Work out the finished part from the listing and answer in its coordinate system (mm). Give positions to 0.01 mm unless a question says otherwise; leave off trailing zeros. Write each loop counter-clockwise with the first axis right and the second up, starting at its lowest first coordinate (ties: lowest second). Pieces come first, ordered by that corner, then holes. Notation, with made-up numbers: (-13.5, 48.25) - (-2.5, 48.25) arc R16 cw to (-2.5, 57.25) - close; hole circle Ø2 at (57.5, -14.75). An arc over 180 degrees is marked (long way). Write item = value, one per line.
from build123d import *

# Parameters (mm, degrees)
SKETCH_1_W             = 295
SKETCH_1_H             = 200
EXTRUDE_1_DEPTH        = 5
SKETCH_2_R             = 1.6
CUT_EXTRUDE_549_DEPTH  = 357.440738412
SKETCH_3_R             = 1.6
CUT_EXTRUDE_902_DEPTH  = 5
SKETCH_4_R             = 1.6
CUT_EXTRUDE_1255_DEPTH = 5
SKETCH_5_R             = 1.6
CUT_EXTRUDE_1670_DEPTH = 5
SKETCH_8_R             = 1.6
CUT_EXTRUDE_2229_DEPTH = 50
SKETCH_10_R            = 1.6
CUT_EXTRUDE_2729_DEPTH = 357.440738412
CUT_EXTRUDE_3337_DEPTH = 10
FILLET_1_R             = 30


with BuildPart() as part:
    # 草图1 → 凸台-拉伸1 (new body)
    with BuildSketch(Plane.XY):
        with Locations((147.5, 100)):
            Rectangle(SKETCH_1_W, SKETCH_1_H)
    extrude(amount=EXTRUDE_1_DEPTH)

    # 草图2 → Cut-Extrude 549 (cut, through all)
    with BuildSketch(Plane.XY.offset(5)):
        with Locations((285, 120)):
            Circle(SKETCH_2_R)
        with Locations(Location((285, 80, 0), (0, 0, 180))):
            Circle(SKETCH_2_R)
    extrude(amount=-CUT_EXTRUDE_549_DEPTH, mode=Mode.SUBTRACT)

    # 草图3 → Cut-Extrude 902 (cut)
    with BuildSketch(Plane.XY.offset(5)):
        with Locations((251, 6.5)):
            Circle(SKETCH_3_R)
        with Locations((212.6, 6.5)):
            Circle(SKETCH_3_R)
        with Locations(Location((44, 6.5, 0), (0, 0, 180))):
            Circle(SKETCH_3_R)
        with Locations(Location((82.4, 6.5, 0), (0, 0, 180))):
            Circle(SKETCH_3_R)
        with Locations(Location((251, 193.5, 0), (0, 0, 180))):
            Circle(SKETCH_3_R)
        with Locations(Location((212.6, 193.5, 0), (0, 0, 180))):
            Circle(SKETCH_3_R)
        with Locations((82.4, 193.5)):
            Circle(SKETCH_3_R)
        with Locations((44, 193.5)):
            Circle(SKETCH_3_R)
    extrude(amount=-CUT_EXTRUDE_902_DEPTH, mode=Mode.SUBTRACT)

    # 草图4 → Cut-Extrude 1255 (cut)
    with BuildSketch(Plane.XY.offset(5)):
        with Locations((196, 124.5)):
            Circle(SKETCH_4_R)
        with Locations((254, 124.5)):
            Circle(SKETCH_4_R)
        with Locations((254, 75.5)):
            Circle(SKETCH_4_R)
        with Locations((196, 75.5)):
            Circle(SKETCH_4_R)
    extrude(amount=-CUT_EXTRUDE_1255_DEPTH, mode=Mode.SUBTRACT)

    # 草图5 → Cut-Extrude 1670 (cut)
    with BuildSketch(Plane.XY.offset(5)):
        with Locations((110.04, 122.5)):
            Circle(SKETCH_5_R)
        with Locations((184.96, 122.5)):
            Circle(SKETCH_5_R)
        with Locations((184.96, 77.5)):
            Circle(SKETCH_5_R)
        with Locations((110.04, 77.5)):
            Circle(SKETCH_5_R)
    extrude(amount=-CUT_EXTRUDE_1670_DEPTH, mode=Mode.SUBTRACT)

    # 草图8 → Cut-Extrude 2229 (cut)
    with BuildSketch(Plane.XY.offset(5)):
        with Locations((154.299232912, 145.494729715)):
            Circle(SKETCH_8_R)
        with Locations(Location((140.700767088, 145.494729715, 0), (0, 0, 180))):
            Circle(SKETCH_8_R)
        with Locations(Location((154.299232912, 54.505270285, 0), (0, 0, 180))):
            Circle(SKETCH_8_R)
        with Locations((140.700767088, 54.505270285)):
            Circle(SKETCH_8_R)
    extrude(amount=-CUT_EXTRUDE_2229_DEPTH, mode=Mode.SUBTRACT)

    # 草图10 → Cut-Extrude 2729 (cut, through all)
    with BuildSketch(Plane.XY.offset(5)):
        with Locations((59.36, 190.7)):
            Circle(SKETCH_10_R)
        with Locations(Location((235.64, 190.7, 0), (0, 0, 180))):
            Circle(SKETCH_10_R)
        with Locations((235.64, 9.3)):
            Circle(SKETCH_10_R)
        with Locations(Location((59.36, 9.3, 0), (0, 0, 180))):
            Circle(SKETCH_10_R)
    extrude(amount=-CUT_EXTRUDE_2729_DEPTH, mode=Mode.SUBTRACT)

    # 草图11 → Cut-Extrude 3337 (cut)
    with BuildSketch(Plane.XY.offset(5)):
        with BuildLine():
            Line((60, 160), (110, 160))
            ThreePointArc((110, 160), (115, 155), (110, 150))
            Line((110, 150), (60, 150))
            ThreePointArc((60, 150), (55, 155), (60, 160))
        make_face()
        with BuildLine():
            Line((60, 40), (110, 40))
            ThreePointArc((110, 40), (115, 45), (110, 50))
            Line((110, 50), (60, 50))
            ThreePointArc((60, 50), (55, 45), (60, 40))
        make_face()
        with BuildLine():
            Line((235, 40), (185, 40))
            ThreePointArc((185, 40), (180, 45), (185, 50))
            Line((185, 50), (235, 50))
            ThreePointArc((235, 50), (240, 45), (235, 40))
        make_face()
        with BuildLine():
            Line((235, 160), (185, 160))
            ThreePointArc((185, 160), (180, 155), (185, 150))
            Line((185, 150), (235, 150))
            ThreePointArc((235, 150), (240, 155), (235, 160))
        make_face()
    extrude(amount=-CUT_EXTRUDE_3337_DEPTH, mode=Mode.SUBTRACT)

    # 圆角1
    fillet_1_edges = [part.edges().sort_by_distance(p)[0] for p in [
        (0, 200, 2.5),
        (295, 200, 2.5),
        (295, 0, 2.5),
        (0, 0, 2.5),
    ]]
    fillet(fillet_1_edges, radius=FILLET_1_R)


solid = part.part
1. Given pin 1 (1 mm diameter, centred on y = 28.5, z = 3.5, fed in from -X), flat-ended and moving along its own axis, determine where the tip first touches the part or whether it passes through.
Solution:
pin_1 = 0.02
2. Find section B-B, the plane z = 3.2. Give the number of separate pieces and of enclosed holes in the cut face, then the cut area to 3 significant figures.
Solution:
separate_pieces = 1
enclosed_holes = 30
area = 55,700 mm^2
3. Find section A-A, the plane x = 68. Give the vertices of the cut face in (y, z), then the cut area to 3 significant figures.
Solution:
outline = (0, 0) - (40, 0) - (40, 5) - (0, 5) - close; (50, 0) - (150, 0) - (150, 5) - (50, 5) - close; (160, 0) - (200, 0) - (200, 5) - (160, 5) - close
area = 900 mm^2
4. Straight lines are drawn through the part: line 1 (Y direction, x = 82.5, z = 0.45); line 2 (Y direction, x = 233, z = 4.55); line 3 (Y direction, x = 285, z = 1). For each, find the intervals that lie inside material, in ascending order.
Solution:
line_1 = 0 to 4.9, 8.1 to 40, 50 to 150, 160 to 191.9, 195.1 to 200
line_2 = 0 to 40, 50 to 150, 160 to 200
line_3 = 7.64 to 78.4, 81.6 to 118.4, 121.6 to 192.36
